from build123d import *

# Parameters (mm, degrees)
SKETCH_1_W                     = 120
SKETCH_1_H                     = 120
EXTRUDE_1_DEPTH                = 5
FILLET_1_R                     = 10
SKETCH_11_R                    = 1
CUT_EXTRUDE_2_DEPTH            = 10
HOLE_WIZARD_M3_1_D             = 3.4
HOLE_WIZARD_M3_1_DEPTH         = 5
HOLE_WIZARD_M3_1_CSINK_D       = 6.6
HOLE_WIZARD_M3_1_CSINK_ANGLE   = 90
HOLE_WIZARD_M3_1_2_OUTLINE_R   = 1.25
HOLE_WIZARD_M3_1_2_DEPTH       = 5
CUT_EXTRUDE_3_REACH            = 87
FILLET_2_R                     = 2
SKETCH_17_OUTSIDE_W            = 155.956
SKETCH_17_OUTSIDE_H            = 155.956
CUT_EXTRUDE_4_DEPTH            = 10
SKETCH_18_R                    = 1.6
SKETCH_18_W                    = 15
SKETCH_18_H                    = 40
EXTRUDE_2_DEPTH                = 5
FILLET_3_R                     = 5
SKETCH_23_R                    = 10
CUT_EXTRUDE_5_DEPTH            = 10
HOLE_WIZARD_M3_1_3_D           = 3.4
HOLE_WIZARD_M3_1_3_DEPTH       = 6
HOLE_WIZARD_M3_1_3_CSINK_D     = 6.4
HOLE_WIZARD_M3_1_3_CSINK_ANGLE = 90
HOLE_WIZARD_M3_1_3_TIP         = 1.021463052
CHAMFER_2_SIZE                 = 0.5


# Read off the part's stored shape, not the designer's step: M3 螺纹孔1
with BuildPart() as part:
    # 草图1 → 凸台-拉伸1 (new body)
    with BuildSketch(Plane(origin=(0, 0, 0), x_dir=(1, 0, 0), z_dir=(0, 1, 0))):
        Rectangle(SKETCH_1_W, SKETCH_1_H)
    extrude(amount=EXTRUDE_1_DEPTH)

    # 圆角1
    fillet_1_edges = [part.edges().sort_by_distance(p)[0] for p in [
        (60, 2.5, 60),
        (-60, 2.5, 60),
        (-60, 2.5, -60),
        (60, 2.5, -60),
    ]]
    fillet(fillet_1_edges, radius=FILLET_1_R)

    # 草图11 → 切除-拉伸2 (cut)
    with BuildSketch(Plane(origin=(0, 5, 0), x_dir=(1, 0, 0), z_dir=(0, 1, 0))):
        with Locations(Location((-13.959899742, 19.214153616, 0), (0, 0, 270))):
            Circle(SKETCH_11_R)
        with Locations(Location((-19.214153616, 13.959899742, 0), (0, 0, 270))):
            Circle(SKETCH_11_R)
        with Locations(Location((19.214153616, 13.959899742, 0), (0, 0, 270))):
            Circle(SKETCH_11_R)
        with Locations(Location((13.959899742, 19.214153616, 0), (0, 0, 270))):
            Circle(SKETCH_11_R)
        with Locations(Location((-19.214153616, -13.959899742, 0), (0, 0, 270))):
            Circle(SKETCH_11_R)
        with Locations(Location((-13.959899742, -19.214153616, 0), (0, 0, 270))):
            Circle(SKETCH_11_R)
        with Locations(Location((19.214153616, -13.959899742, 0), (0, 0, 270))):
            Circle(SKETCH_11_R)
        with Locations(Location((13.959899742, -19.214153616, 0), (0, 0, 270))):
            Circle(SKETCH_11_R)
    extrude(amount=-CUT_EXTRUDE_2_DEPTH, mode=Mode.SUBTRACT)

    # Hole Wizard M3 _1
    with Locations(Plane(origin=(0, 0, 0), x_dir=(-1, 0, 0), z_dir=(0, -1, 0))):
        with Locations((-13.959899742, 19.214153616), (-19.214153616, 13.959899742), (-19.214153616, -13.959899742), (-13.959899742, -19.214153616), (13.959899742, -19.214153616), (19.214153616, -13.959899742), (13.959899742, 19.214153616), (19.214153616, 13.959899742)):
            CounterSinkHole(HOLE_WIZARD_M3_1_D / 2, HOLE_WIZARD_M3_1_CSINK_D / 2, depth=HOLE_WIZARD_M3_1_DEPTH, counter_sink_angle=HOLE_WIZARD_M3_1_CSINK_ANGLE)

    # Hole Wizard M3 _1 2 outline → Hole Wizard M3 _1 2 (cut)
    with BuildSketch(Plane(origin=(0, 0, 0), x_dir=(1, 0, 0), z_dir=(0, 1, 0))):
        with Locations((-25.986174209, -25.986174209)):
            Circle(HOLE_WIZARD_M3_1_2_OUTLINE_R)
        with Locations((25.986174209, -25.986174209)):
            Circle(HOLE_WIZARD_M3_1_2_OUTLINE_R)
        with Locations((25.986174209, 25.986174209)):
            Circle(HOLE_WIZARD_M3_1_2_OUTLINE_R)
        with Locations((-25.986174209, 25.986174209)):
            Circle(HOLE_WIZARD_M3_1_2_OUTLINE_R)
    extrude(amount=HOLE_WIZARD_M3_1_2_DEPTH, mode=Mode.SUBTRACT)

    # 草图16 → 切除-拉伸3 (cut, up to next)
    with BuildSketch(Plane(origin=(0, 5, 0), x_dir=(1, 0, 0), z_dir=(0, 1, 0)), mode=Mode.PRIVATE) as cut_extrude_3_sk1:
        Polygon((0, -24.5), (14, -24.5), (17.5, -40.5), (0, -40.5), (-17.5, -40.5), (-14, -24.5), align=None)
    cut_extrude_3_tool1 = extrude(cut_extrude_3_sk1.sketch, amount=-CUT_EXTRUDE_3_REACH, mode=Mode.PRIVATE) & part.part
    add(cut_extrude_3_tool1.solids().sort_by_distance((0, 5, 32.796296))[0], mode=Mode.SUBTRACT)

    # 圆角2
    fillet_2_edges = [part.edges().sort_by_distance(p)[0] for p in [
        (-14, 2.5, 24.5),
        (14, 2.5, 24.5),
        (17.5, 2.5, 40.5),
        (-17.5, 2.5, 40.5),
    ]]
    fillet(fillet_2_edges, radius=FILLET_2_R)

    # 草图17 outside → 切除-拉伸4 (cut)
    with BuildSketch(Plane(origin=(0, 5, 0), x_dir=(1, 0, 0), z_dir=(0, 1, 0))):
        Rectangle(SKETCH_17_OUTSIDE_W, SKETCH_17_OUTSIDE_H)
        with BuildLine():
            Line((1e-09, -46.5), (-38, -46.5))
            ThreePointArc((-38, -46.5), (-46.485281374, -42.985281374), (-50, -34.5))
            Line((-50, -34.5), (-50, 34.5))
            ThreePointArc((-50, 34.5), (-46.485281374, 42.985281374), (-38, 46.5))
            Line((-38, 46.5), (1e-09, 46.5))
            ThreePointArc((1e-09, 46.5), (46.5, 0), (1e-09, -46.5))
        make_face(mode=Mode.SUBTRACT)
    extrude(amount=-CUT_EXTRUDE_4_DEPTH, mode=Mode.SUBTRACT)

    # 草图18 → 凸台-拉伸2 (add)
    # profile 1 of 2: a face of its own
    with BuildSketch(Plane(origin=(0, 5, 0), x_dir=(1, 0, 0), z_dir=(0, 1, 0))):
        with BuildLine():
            Line((65, 20), (65, -20))
            Line((65, -20), (41.979161497, -20))
            ThreePointArc((41.979161497, -20), (46.5, 0), (41.979161497, 20))
            Line((41.979161497, 20), (65, 20))
        make_face()
        with Locations(Location((60, 15, 0), (0, 0, 270))):
            Circle(SKETCH_18_R, mode=Mode.SUBTRACT)
        with Locations(Location((60, -15, 0), (0, 0, 270))):
            Circle(SKETCH_18_R, mode=Mode.SUBTRACT)
    # profile 2 of 2: a face of its own
    with BuildSketch(Plane(origin=(0, 5, 0), x_dir=(1, 0, 0), z_dir=(0, 1, 0))):
        with Locations((-57.5, 0)):
            Rectangle(SKETCH_18_W, SKETCH_18_H)
        with Locations(Location((-60, 15, 0), (0, 0, 270))):
            Circle(SKETCH_18_R, mode=Mode.SUBTRACT)
        with Locations(Location((-60, -15, 0), (0, 0, 270))):
            Circle(SKETCH_18_R, mode=Mode.SUBTRACT)
    extrude(amount=-EXTRUDE_2_DEPTH)

    # 圆角3
    fillet_3_edges = [part.edges().sort_by_distance(p)[0] for p in [
        (-50, 2.5, 20),
        (-65, 2.5, 20),
        (-65, 2.5, -20),
        (-50, 2.5, -20),
        (65, 2.5, 20),
        (41.979161497, 2.5, 20),
        (41.979161497, 2.5, -20),
        (65, 2.5, -20),
    ]]
    fillet(fillet_3_edges, radius=FILLET_3_R)

    # 草图23 → 切除-拉伸5 (cut)
    with BuildSketch(Plane.XZ):
        with Locations(Location((0, 0, 0), (0, 0, 270))):
            Circle(SKETCH_23_R)
    extrude(amount=-CUT_EXTRUDE_5_DEPTH, mode=Mode.SUBTRACT)

    # Hole Wizard M3 _1 3
    with Locations(Plane(origin=(0, 5, 0), x_dir=(1, 0, 0), z_dir=(0, 1, 0))):
        with Locations((-60, 15), (-60, -15), (60, 15), (60, -15)):
            CounterSinkHole(HOLE_WIZARD_M3_1_3_D / 2, HOLE_WIZARD_M3_1_3_CSINK_D / 2, depth=HOLE_WIZARD_M3_1_3_DEPTH, counter_sink_angle=HOLE_WIZARD_M3_1_3_CSINK_ANGLE)
            with Locations((0, 0, -(HOLE_WIZARD_M3_1_3_DEPTH + HOLE_WIZARD_M3_1_3_TIP / 2))):  # 118° drill point
                Cone(0, HOLE_WIZARD_M3_1_3_D / 2, HOLE_WIZARD_M3_1_3_TIP, mode=Mode.SUBTRACT)

    # 倒角2
    chamfer_2_edges = [part.edges().sort_by_distance(p)[0] for p in [
        (0, 0, 40.5),
        (0, 5, 40.5),
        (-15.656507616, 0, 32.072606242),
        (-15.656507616, 5, 32.072606242),
        (15.656507616, 0, 32.072606242),
        (15.656507616, 5, 32.072606242),
        (0, 0, 24.5),
        (0, 5, 24.5),
        (-16.573217131, 5, 39.754035981),
        (-16.573217131, 0, 39.754035981),
        (16.573217131, 5, 39.754035981),
        (16.573217131, 0, 39.754035981),
        (13.644243562, 5, 24.94199045),
        (13.644243562, 0, 24.94199045),
        (-13.644243562, 5, 24.94199045),
        (-13.644243562, 0, 24.94199045),
        (23.58616202, 0, 40.07421816),
        (-19, 5, 46.5),
        (-46.485281374, 5, 42.985281374),
        (-50, 0, -29.75),
        (-46.485281374, 0, -42.985281374),
        (-19, 0, -46.5),
        (-19, 0, 46.5),
        (-46.485281374, 0, 42.985281374),
        (23.58616202, 5, 40.07421816),
        (-19, 5, -46.5),
        (-46.485281374, 5, -42.985281374),
        (-50, 5, -29.75),
        (-57.5, 0, -20),
        (-57.5, 5, -20),
        (52.51249653, 5, 20),
        (65, 5, 0),
        (52.51249653, 5, -20),
        (23.58616202, 5, -40.07421816),
        (-65, 5, 0),
        (-57.5, 5, 20),
        (-50, 5, 29.75),
        (63.535533906, 5, -18.535533906),
        (63.535533906, 5, 18.535533906),
        (-63.535533906, 5, 18.535533906),
        (-63.535533906, 5, -18.535533906),
        (-65, 0, 0),
        (-50, 0, 29.75),
        (-57.5, 0, 20),
        (23.58616202, 0, -40.07421816),
        (52.51249653, 0, -20),
        (65, 0, 0),
        (52.51249653, 0, 20),
        (63.535533906, 0, -18.535533906),
        (63.535533906, 0, 18.535533906),
        (-63.535533906, 0, 18.535533906),
        (-63.535533906, 0, -18.535533906),
        (-51.464466094, 5, -21.464466094),
        (-51.464466094, 0, -21.464466094),
        (-51.464466094, 5, 21.464466094),
        (-51.464466094, 0, 21.464466094),
        (42.488846606, 5, 20.690944284),
        (42.488846606, 0, 20.690944284),
        (42.488846606, 5, -20.690944284),
        (42.488846606, 0, -20.690944284),
        (0, 5, 10),
        (0, 0, 10),
    ]]
    chamfer(chamfer_2_edges, length=CHAMFER_2_SIZE)


solid = part.part
Part model, mm, in its own coordinate system. A direction names the side the tool comes from. Round coordinates to 2 decimals unless told otherwise and drop trailing zeros. Order: outer loops, then holes, each group sorted by start corner. A loop starts at its lowest first (then second) coordinate and runs counter-clockwise, first axis right, second up. Notation, with made-up numbers: (59.5, 49.25) -> (111.5, 49.25) arc R26 cw to (111.5, 71.25) -> close; hole circle Ø6 at (13, 7.5). An arc over 180 degrees is marked (long way). Put each result on its own line as item: value.
Q1. Band-saw the part on A-A (z = 0). Give the cut face in (x, y).
From the geometry:
outline: (-65, 0.5) -> (-64.5, 0) -> (-10.5, 0) -> (-10, 0.5) -> (-10, 4.5) -> (-10.5, 5) -> (-64.5, 5) -> (-65, 4.5) -> close; (10, 0.5) -> (10.5, 0) -> (64.5, 0) -> (65, 0.5) -> (65, 4.5) -> (64.5, 5) -> (10.5, 5) -> (10, 4.5) -> close
Q2. Wall check: line 1 (Z direction, x = 59, y = 2.4); line 2 (Z direction, x = 18, y = 3.65); line 3 (X direction, y = 0.2, z = -13). Give the ranges that are in metal, low to high. Write a range as [from, to].
From the geometry:
line 1: z = [-20, -16.37], [-13.63, 13.63], [16.37, 20]
line 2: z = [-42.87, -15.15], [-12.77, 12.77], [15.15, 42.87]
line 3: x = [-64.7, -22.16], [-16.27, 16.27], [22.16, 64.7]
Q3. Band-saw the part on B-B (x = 4). State how many separate pieces and enclosed holes the cut face has, and give its area (3 significant figures).
From the geometry:
separate pieces: 3
enclosed holes: 0
area: 290 mm2
Q4. Tool access for faces 5 (the face through (-51.409, 4.635, -21.329)), 6 (the face through (-16.59, 2.47, 39.73)), 7 (the face through (-16.662, 0.365, 39.86)): list every direction of +Z, -Z, +X, -X, +Y, -Y with a clear straight run to the whole face (end or side of a thin tool).
From the geometry:
face 5: -Z, -X, +Y
face 6: +Y, -Y
face 7: -Y
Q5. Pin check, flat tips, straight feed: pin 1 Ø2.5 at (x, z) = (19.21, 13.96) entering from +Y; pin 2 Ø1.2 at (y, z) = (3.5, -29.5) entering from -X; pin 3 Ø5.5 at (x, z) = (13.96, -19.21) entering from -Y; pin 4 Ø2 at (x, y) = (-58, 3) entering from -Z. Stop position of each tip, or through.
From the geometry:
pin 1: passes through
pin 2: stops at x = -50
pin 3: stops at y = 0.55
pin 4: stops at z = -20
Q6. Pull direction Z, two halves, no side cores. Call faces 1 (the face through (-64, 2, -18)), 2 (the face through (17.865, 3.324, 14.994)), 3 (the face through (-63.246, 4.858, 18.319)), 4 (the face through (-1, 5, -11)): pulls with the +Z half, pulls with the -Z half, needs draft (parallel to the pull), parting line crosses it, or undercut.
From the geometry:
face 1: pulls with the -Z half
face 2: undercut
face 3: pulls with the +Z half
face 4: needs draft
